Geometry check sheet. Reference: the model listing, model coordinates, mm. A direction names the side the tool comes from. Round coordinates to 2 decimals unless told otherwise and drop trailing zeros. Loops run counter-clockwise (first coordinate to the right, second up) from the corner with the lowest first, then second, coordinate; pieces in that order, holes last.
```python
from build123d import *

# Parameters (mm, degrees)
F1_DEPTH = 63.5
F0_W     = 25.4
F0_H     = 19.05
F2_DEPTH = 25.4
F3_DEPTH = 7.9375


with BuildPart() as f1:
    # F0 (on Front) → F1 (new body, symmetric)
    with BuildSketch(Plane.XZ):
        Polygon((-41.275, -9.525), (41.275, -9.525), (41.275, 9.525), (22.225, 9.525), (-41.275, 9.525), align=None)
    extrude(amount=F1_DEPTH, both=True)

    # F0 (on Front) → F2 (join, symmetric)
    with BuildSketch(Plane.XZ):
        with BuildLine():
            Line((22.225, 9.525), (41.275, 9.525))
            Line((41.275, 9.525), (41.275, 26.9875))
            ThreePointArc((41.275, 26.9875), (45.9246798487, 38.2128201513), (57.15, 42.8625))
            Line((57.15, 42.8625), (60.325, 42.8625))
            Line((60.325, 42.8625), (60.325, 61.9125))
            Line((60.325, 61.9125), (57.15, 61.9125))
            ThreePointArc((57.15, 61.9125), (32.4542956671, 51.6832043329), (22.225, 26.9875))
            Line((22.225, 26.9875), (22.225, 9.525))
        make_face()
        with Locations((73.025, 52.3875)):
            Rectangle(F0_W, F0_H)
        Polygon((85.725, 66.675), (85.725, 61.9125), (85.725, 42.8625), (85.725, 38.1), (111.125, 38.1), (111.125, 66.675), align=None)
    extrude(amount=F2_DEPTH, both=True)

    # F0 (on Front) → F3 (join, symmetric)
    with BuildSketch(Plane.XZ):
        with BuildLine():
            add(Edge.make_bspline(
                [(-41.275, 9.525), (-41.275, 38.2137889473), (10.6306826578, 61.9125), (57.15, 61.9125)],
                knots=[0, 0, 0, 0, 111.4985685166, 111.4985685166, 111.4985685166, 111.4985685166], degree=3))
            Line((-41.275, 9.525), (22.225, 9.525))
            Line((22.225, 9.525), (22.225, 26.9875))
            ThreePointArc((22.225, 26.9875), (32.4542956671, 51.6832043329), (57.15, 61.9125))
        make_face()
    extrude(amount=F3_DEPTH, both=True)


solid = f1.part
```
1) Sectioned sample at C-C, the plane y = -42. Record the cut outline in (x, z) (3 decimals), then the cut area to 3 significant figures.
Report:
outline: (-41.275, -9.525) - (41.275, -9.525) - (41.275, 9.525) - (-41.275, 9.525) - close
area: 1,570 mm2
2) Gauge pin test, flat ends, axial feed: pin 1 (1.5 mm diameter, centred on x = 71, y = -26, fed in from -Z); pin 2 (1 mm diameter, centred on x = 76.5, y = 5.5, fed in from +Z); pin 3 (17 mm diameter, centred on x = 83, z = 46.5, fed in from +Y). Record the tip position at first contact, or that the pin passes through.
Report:
pin 1: stops at z = 42.86
pin 2: stops at z = 61.91
pin 3: stops at y = 25.4
3) Sectioned sample at B-B, the plane z = -4. Record the cut outline in (x, y) (3 decimals), then the cut area to 3 significant figures.
Report:
outline: (-41.275, -63.5) - (41.275, -63.5) - (41.275, 63.5) - (-41.275, 63.5) - close
area: 10,500 mm2
4) Access from +Z, -Z, +X, -X, +Y, -Y to the whole of each face (thin tool, end or side, straight path). Record for faces 1 (the face through (32.727, -16.791, 51.953)), 2 (the face through (45.802, -0.356, 38.089)), 3 (the face through (32.727, 16.547, 51.953)), 4 (the face through (66, -25.4, 45)), 5 (the face through (66, 25.4, 45)).
Report:
face 1: +Z, -X, -Y
face 2: -Z, +Y, -Y
face 3: +Z, -X, +Y
face 4: +Z, +X, -X, -Y
face 5: +Z, +X, -X, +Y
5) Scan lines: line 1 along Z through (x, y) = (93, -24) (3 decimals); line 2 along X through (y, z) = (-48, -3.5) (3 decimals); line 3 along Y through (x, z) = (73, 48). Record each from-to range of solid material in increasing order.
Report:
line 1: z = 38.1 to 66.675
line 2: x = -41.275 to 41.275
line 3: y = -25.4 to 25.4
